Source: CAD feature listing. Evaluate the final solid. Frame: model axes, mm. Face numbers are marked on the shaded views. Give positions to 0.01 mm unless a question says otherwise; leave off trailing zeros. Loops run counter-clockwise (first coordinate to the right, second up) from the corner with the lowest first, then second, coordinate; pieces in that order, holes last. Notation, with made-up numbers: (29, -35) -> (73, -35) arc R34 ccw to (73, 1) -> close; hole circle Ø9 at (-24, -32). An arc over 180 degrees is marked (long way). Return JSON: item names as keys, results as strings. Group by question number.
(1) Cut plane A-A on x = 0. Return loops of the section in (y, z) (3 decimals), then the cut area to 3 significant figures.
(2) Cut plane C-C on y = 3.25. Return loops of the section in (x, z), then the cut area to 3 significant figures.
(3) Draft query along Z for the marked faces 1, 2 and 3. Return one class per face: released by +Z, released by -Z, zero draft, split by the parting line, or undercut.
(4) Ray query, line 1 (Z direction, x = 0, y = -0.75); line 2 (X direction, y = -3, z = 36); line 3 (Z direction, x = 0.5, y = -0.5). Return the intervals inside material, ascending. Write a range as from..to.
(5) Cut plane B-B on z = 3. Return loops of the section in (x, y) (3 decimals), then the cut area to 3 significant figures.
```python
from build123d import *

# Parameters (mm, degrees)
ESQUISSE1_W                     = 10
ESQUISSE1_H                     = 10
BOSS_EXTRU_1_DEPTH              = 54.8
BOSS_EXTRU_1_DEPTH_BACK         = 2
TROU_TARAUD_M3X0_51_D           = 2.5
TROU_TARAUD_M3X0_51_CSINK_D     = 3.05
TROU_TARAUD_M3X0_51_CSINK_ANGLE = 90


with BuildPart() as part:
    # Esquisse1 → Boss.-Extru.1 (new body, two sides)
    with BuildSketch(Plane.XY) as boss_extru_1_sk:
        Rectangle(ESQUISSE1_W, ESQUISSE1_H)
    extrude(amount=BOSS_EXTRU_1_DEPTH)
    extrude(boss_extru_1_sk.sketch, amount=-BOSS_EXTRU_1_DEPTH_BACK)

    # Trou taraud_ M3x0.51 (through all)
    with Locations(Plane(origin=(0, 5, 0), x_dir=(1, 0, 0), z_dir=(0, 1, 0))):
        with Locations((0, -36), (0, -3)):
            CounterSinkHole(TROU_TARAUD_M3X0_51_D / 2, TROU_TARAUD_M3X0_51_CSINK_D / 2, counter_sink_angle=TROU_TARAUD_M3X0_51_CSINK_ANGLE)


solid = part.part
```
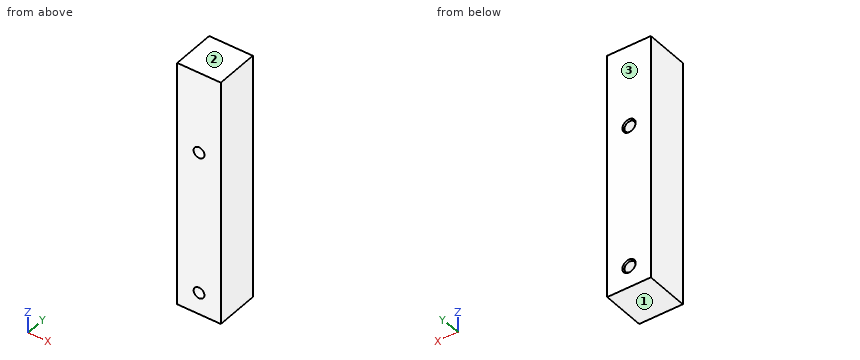
Answers:
{
 "1": {"outline": "(-5, -2) -> (5, -2) -> (5, 1.475) -> (4.725, 1.75) -> (-5, 1.75) -> close; (-5, 4.25) -> (4.725, 4.25) -> (5, 4.525) -> (5, 34.475) -> (4.725, 34.75) -> (-5, 34.75) -> close; (-5, 37.25) -> (4.725, 37.25) -> (5, 37.525) -> (5, 54.8) -> (-5, 54.8) -> close", "area": "518 mm²"},
 "2": {"outline": "(-5, -2) -> (5, -2) -> (5, 54.8) -> (-5, 54.8) -> close; hole circle Ø2.5 at (0, 3); hole circle Ø2.5 at (0, 36)", "area": "558 mm²"},
 "3": {"face 1": "released by -Z", "face 2": "released by +Z", "face 3": "zero draft"},
 "4": {"line 1": "-2..1.75, 4.25..34.75, 37.25..54.8", "line 2": "-5..-1.25, 1.25..5", "line 3": "-2..1.85, 4.15..34.85, 37.15..54.8"},
 "5": {"outline": "(-5, -5) -> (-1.25, -5) -> (-1.25, 4.725) -> (-1.525, 5) -> (-5, 5) -> close; (1.25, -5) -> (5, -5) -> (5, 5) -> (1.525, 5) -> (1.25, 4.725) -> close", "area": "74.9 mm²"}
}
